Design review of the part built by this model. Coordinates are the model's own, in mm. A direction names the side the tool comes from. Coordinates: 2 decimals unless noted, no trailing zeros. Loops run counter-clockwise (first coordinate to the right, second up) from the corner with the lowest first, then second, coordinate; pieces in that order, holes last. Notation, with made-up numbers: (80, -39) -> (133, -39) arc R16 ccw to (133, -28) -> close; hole circle Ø11 at (-9, 31.25). An arc over 180 degrees is marked (long way). Use CSV: the item, a comma, the result in double quotes.
Autodesk Inventor part; units mm, degrees
ref_plane "Start Plane" through (0, 0, 80) normal (0, 0, 1) x (1, 0, 0)
ref_plane "End Plane" through (0, 0, 2770) normal (0, 0, 1) x (1, 0, 0)
ref_plane "YZ Plane" through (0, 0, 0) normal (1, 0, 0) x (0, 1, 0)
ref_plane "Start Plane" through (0, 0, 80) normal (0, 0, 1) x (1, 0, 0)
ref_plane "End Plane" through (0, 0, 2770) normal (0, 0, 1) x (1, 0, 0)
sketch "Sketch" plane through (0, 0, 0) normal (0, 0, 1) x (1, 0, 0)
  line L0 (-40, -34) -> (-40, 34)
  line L1 (-34, 40) -> (34, 40)
  line L2 (40, 34) -> (40, -34)
  line L3 (34, -40) -> (-34, -40)
  arc A0 (-40, -34) -> (-34, -40) centre (-34, -34) ccw
  arc A1 (40, 34) -> (34, 40) centre (34, 34) ccw
  arc A2 (-34, 40) -> (-40, 34) centre (-34, 34) ccw
  arc A3 (34, -40) -> (40, -34) centre (34, -34) ccw
  arc A4 (-34, 37) -> (-37, 34) centre (-34, 34) ccw
  line L4 (-34, 37) -> (34, 37)
  arc A5 (37, 34) -> (34, 37) centre (34, 34) ccw
  line L5 (37, 34) -> (37, -34)
  arc A6 (34, -37) -> (37, -34) centre (34, -34) ccw
  line L6 (34, -37) -> (-34, -37)
  arc A7 (-37, -34) -> (-34, -37) centre (-34, -34) ccw
  line L7 (-37, -34) -> (-37, 34)
  line L8 (0, 57.7397) -> (0, -57.7397) construction
  line L9 (-57.7397, 0) -> (57.7397, 0) construction
  dimension "d7" = 6
  dimension "d9" = 80
  dimension "d11" = 80
  dimension "d12" = 3
  dimension "d15" = 40
  dimension "d16" = 40
extrude "Body" add sketch "Sketch" along normal up to surface (2690 mm away) from surface at 80
sketch "Sketch3" plane through (0, 0, 0) normal (0, 0, 1) x (1, 0, 0)
  line L0 (0, 0) -> (10, 0)
ref_plane "Work Plane3" through (0, 0, 0) normal (0, -1, 0) x (1, 0, 0)
sketch "Sketch4" plane through (0, 0, 0) normal (0, -1, 0) x (1, 0, 0)
  line L0 (-2, 80) -> (12, 80)
  line L1 (-2, 2770) -> (12, 2770)
  dimension "d18" = 2690
equation "\"d7\" = G_IR"
equation "\"d9\" = G_W"
equation "\"d11\" = G_H"
equation "\"d12\" = G_T"
equation "\"d15\" = 0.5 * d9"
equation "\"d16\" = 0.5 * d11"
equation "\"d3\" = G_L"
equation "\"G_W\" = 80"
equation "\"G_H\" = 80"
equation "\"G_T\" = 3"
equation "\"G_IR\" = 6"
equation "\"G_L\" = d18"
properties part number "ISO 4019 - 80x80x3 - 2690" material "Steel, Mild"
Item 1: Add section A-A (y = -12.5). Give the boundary of the cut face in (x, z), then the cut area to 3 significant figures.
Checked values:
outline,"(-40, 80) -> (-37, 80) -> (-37, 2770) -> (-40, 2770) -> close; (37, 80) -> (40, 80) -> (40, 2770) -> (37, 2770) -> close"
area,"16,100 mm^2"
Item 2: Machinability: for faces 5 (the face through (37, 0, 1406)), 6 (the face through (40, 0, 1406)), which of the approach directions +Z, -Z, +X, -X, +Y, -Y give a long, thin tool a straight path to every point of the face, cutting with its end or side? Answer none if there is none.
Checked values:
face 5,"+Z, -Z"
face 6,"+Z, -Z, +X, +Y, -Y"
Item 3: Draft analysis for pull direction Y (two halves, no side actions). For faces 1 (the face through (0, -40, 1406)), 2 (the face through (0, -37, 1406)), 3 (the face through (0, 37, 1406)), 4 (the face through (0, 39, 80)), state which applies: pulls with the +Y half, pulls with the -Y half, needs draft (parallel to the pull), parting line crosses it, or undercut.
Checked values:
face 1,"pulls with the -Y half"
face 2,"undercut"
face 3,"undercut"
face 4,"needs draft"
Item 4: Add section B-B (z = 1442.5). Give the boundary of the cut face in (x, y).
Checked values:
outline,"(-40, -34) arc R6 ccw to (-34, -40) -> (34, -40) arc R6 ccw to (40, -34) -> (40, 34) arc R6 ccw to (34, 40) -> (-34, 40) arc R6 ccw to (-40, 34) -> close; hole (-37, -34) arc R3 ccw to (-34, -37) -> (34, -37) arc R3 ccw to (37, -34) -> (37, 34) arc R3 ccw to (34, 37) -> (-34, 37) arc R3 ccw to (-37, 34) -> close"
Item 5: To check wall thickness, follow line 1 along X through (y, z) = (27, 2577); line 2 along X through (y, z) = (35, 2316.5). State the ranges of each line that lie inside material, in increasing order.
Checked values:
line 1,"-40 to -37, 37 to 40"
line 2,"-39.92 to -36.83, 36.83 to 39.92"
